Read the model definition and answer for the solid it produces. Units are mm, in the model's axes. Face numbers are marked on the shaded views. A direction names the side the tool comes from. Coordinates: 2 decimals unless noted, no trailing zeros. Order: outer loops, then holes, each group sorted by start corner. A loop starts at its lowest first (then second) coordinate and runs counter-clockwise, first axis right, second up. Notation, with made-up numbers: (-16.75, -9) - (35.25, -9) arc R17 ccw to (35.25, 16) - close; hole circle Ø1 at (-34.5, 56.25). An arc over 180 degrees is marked (long way). Use one line per item in the form item = value.
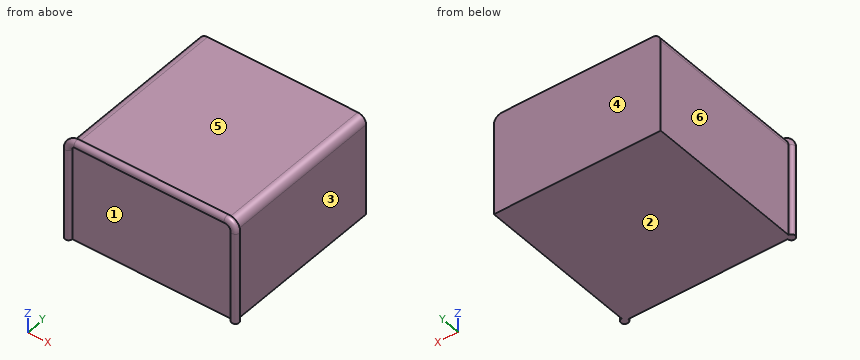
```python
from build123d import *

# Parameters (mm, degrees)
F0_W     = 1000
F0_H     = 600
F1_DEPTH = 1000
F2_R     = 50
F3_R     = 50


with BuildPart() as f1:
    # F0 (on Front) → F1 (new body)
    with BuildSketch(Plane.XZ):
        with Locations((66.8085864745, -99.2259835054)):
            Rectangle(F0_W, F0_H)
    extrude(amount=F1_DEPTH)

    # F2
    f2_edges = [f1.edges().sort_by_distance(p)[0] for p in [
        (-433.191414, -500, 200.774016),
    ]]
    fillet(f2_edges, radius=F2_R)

    # F3
    f3_edges = [f1.edges().sort_by_distance(p)[0] for p in [
        (566.808586, -500, 200.774016),
    ]]
    fillet(f3_edges, radius=F3_R)

    # F5: sweep along a path in F5_path
    with BuildLine(Plane(origin=(-433.1914135255, -1000, -399.2259835054), x_dir=(0, 0, 1), z_dir=(0, -1, 0))) as f5_path:
        Line((0, 0), (550, 0))
        ThreePointArc((550, 0), (585.3553390593, -14.6446609407), (600, -50))
        Line((600, -50), (600, -950))
        ThreePointArc((600, -950), (585.3553390593, -985.3553390593), (550, -1000))
        Line((550, -1000), (0, -1000))
    # F4 (on face) → F5 (sweep)
    with BuildSketch(Plane(origin=(0, 0, -399.2259835054), x_dir=(1, 0, 0), z_dir=(0, 0, -1))):
        with BuildLine():
            ThreePointArc((-433.1914135255, 977.6715629095), (-417.4028242455, 984.21141072), (-410.862976435, 1000))
            Line((-410.862976435, 1000), (-433.1914135255, 1000))
            Line((-433.1914135255, 1000), (-433.1914135255, 977.6715629095))
        make_face()
        with BuildLine():
            Line((-433.1914135255, 1000), (-410.862976435, 1000))
            ThreePointArc((-410.862976435, 1000), (-448.9800028055, 1015.78858928), (-433.1914135255, 977.6715629095))
            Line((-433.1914135255, 977.6715629095), (-433.1914135255, 1000))
        make_face()
    sweep(path=f5_path.line)


solid = f1.part
```
(1) Section A-A, the plane z = 96.5 is taken. Write down the section's boundary in (x, y), then the cut area to 3 significant figures.
Answer list:
outline = (-433.19, -977.67) arc R22.33 ccw (long way) to (-410.86, -1000) - (544.48, -1000) arc R22.33 ccw (long way) to (566.81, -977.67) - (566.81, 0) - (-433.19, 0) - close
area = 1,000,000 mm2
(2) The mould has two halves that part along X. Classify the marked faces 1, 2 and 3: +X half, -X half, draft (parallel to the pull), parting line (faces both ways), or undercut.
Answer list:
face_1 = undercut
face_2 = draft
face_3 = +X half
(3) Straight lines are drawn through the part: L1, parallel to Y at x = 163, z = 135; L2, parallel to Z at x = -128, y = -261; L3, parallel to X at y = -562, z = -232. For each, find the intervals that lie inside material, in ascending order.
Answer list:
L1 = -1000 to 0
L2 = -399.23 to 200.77
L3 = -433.19 to 566.81
(4) Given pin 1 Ø8 at (x, y) = (338.5, -547) entering from +Z; pin 2 Ø12 at (y, z) = (-566, 70) entering from +X; pin 3 Ø4 at (y, z) = (-830, 25) entering from -X, each flat-ended and moving along its own axis, determine where each tip first touches the part or whether it passes through.
Answer list:
pin_1 = 200.77
pin_2 = 566.81
pin_3 = -433.19
(5) Section B-B, the plane y = -637 is taken. Write down the section's boundary in (x, z), then the cut area to 3 significant figures.
Answer list:
outline = (-433.19, -399.23) - (566.81, -399.23) - (566.81, 150.77) arc R50 ccw to (516.81, 200.77) - (-383.19, 200.77) arc R50 ccw to (-433.19, 150.77) - close
area = 599,000 mm2
(6) Section C-C, the plane x = -187 is taken. Write down the section's boundary in (y, z).
Answer list:
outline = (-1000, -399.23) - (0, -399.23) - (0, 200.77) - (-977.67, 200.77) arc R22.33 ccw (long way) to (-1000, 178.45) - close
(7) Which of the six approach directions +Z, -Z, +X, -X, +Y, -Y give full straight-line access (tool end or side, diameter ignored) to the marked faces 4, 5 and 6?
Answer list:
face_4 = +Z, -Z, +X, -X, +Y
face_5 = +Z, +X, -X, +Y
face_6 = +Z, -Z, -X, +Y
